Here's how the part is built. I have some questions about the finished solid (model axes, mm). A direction names the side the tool comes from. Coordinates: 2 decimals unless noted, no trailing zeros. Loops run counter-clockwise (first coordinate to the right, second up) from the corner with the lowest first, then second, coordinate; pieces in that order, holes last. Notation, with made-up numbers: M 54.25,56 L 68.25,56 A29 cw 68.25,87 Z; hole C 27.25,-13.75 d11. An arc over 180 degrees is marked long. Use CSV: the item, a comma, the result in double quotes. Start each with the question number.
Q1. Please list where these lines run through material, in increasing order: probe 1 along Y at (x, z) = (122, 3.05); probe 2 along Y at (x, z) = (144, 11); probe 3 along Y at (x, z) = (182, 16). Write a range as [from, to].
Q2. For pin 1 Ø4 at (y, z) = (91.5, 4) entering from +X; pin 2 Ø6.5 at (x, y) = (74, 48.5) entering from +Z; pin 3 Ø4 at (y, z) = (23.5, 3.5) entering from -X; pin 4 Ø3 at (y, z) = (23, 7) entering from +X, each with a flat end and sliding along its axis, tell me the tip position at first contact or that it passes through.
Q3. Which directions (+Z, -Z, +X, -X, +Y, -Y) give clear straight access to the entire face, cutting with the end or side of a thin tool? Please do faces 1 (the flat face through (243, 107, 4)), 2 (the flat face through (173, 29, 4)).
Q4. If we section it at B-B (x = 32): Please give me the cut outline in (y, z), and give its area (3 significant figures).
Q5. If we section it at A-A (x = 159): Please give me the cut outline in (y, z).
from build123d import *

# Parameters (mm, degrees)
F1_DEPTH = 4
F0_R     = 3
F0_R_2   = 2.5
F0_R_3   = 2
F0_R_4   = 12
F0_R_5   = 8
F2_DEPTH = 8
F3_DEPTH = 30


with BuildPart() as f1:
    # F0 (on Top) → F1 (new body)
    with BuildSketch(Plane.XY):
        with BuildLine():
            Line((236, 122), (236, 77))
            Line((236, 77), (249.9140349643, 77))
            Line((249.9140349643, 77), (286.1814989821, 119.8615483846))
            ThreePointArc((286.1814989821, 119.8615483846), (280.1803788328, 120.1541279906), (278.7929977309, 126))
            Line((278.7929977309, 126), (150, 126))
            Line((150, 126), (150, 122))
            Line((150, 122), (236, 122))
        make_face()
    extrude(amount=F1_DEPTH)



with BuildPart() as f1b:
    # F0 (on Top) → F1, piece 2 (new body)
    with BuildSketch(Plane.XY):
        Polygon((220.2986503489, 42), (243.1448041951, 69), (195, 69), (195, 42), align=None)
    extrude(amount=F1_DEPTH)


with BuildPart() as f1c:
    # F0 (on Top) → F1, piece 3 (new body)
    with BuildSketch(Plane.XY):
        Polygon((203.3755734259, 22), (215.221727272, 36), (177, 36), (177, 22), align=None)
    extrude(amount=F1_DEPTH)


with BuildPart() as f1d:
    # F0 (on Top) → F1, piece 4 (new body)
    with BuildSketch(Plane.XY):
        Polygon((188.1448041951, 4), (199.9909580413, 18), (177, 18), (177, 4), align=None)
    extrude(amount=F1_DEPTH)


with BuildPart() as f1e:
    # F0 (on Top) → F1, piece 5 (new body)
    with BuildSketch(Plane.XY):
        with BuildLine():
            Line((146, 10.582575695), (146, 119.417424305))
            ThreePointArc((146, 119.417424305), (140.4644660941, 120.4644660941), (139.417424305, 126))
            Line((139.417424305, 126), (10.582575695, 126))
            ThreePointArc((10.582575695, 126), (9.5355339059, 120.4644660941), (4, 119.417424305))
            Line((4, 119.417424305), (4, 10.582575695))
            ThreePointArc((4, 10.582575695), (9.5355339059, 9.5355339059), (10.582575695, 4))
            Line((10.582575695, 4), (139.417424305, 4))
            ThreePointArc((139.417424305, 4), (140.4644660941, 9.5355339059), (146, 10.582575695))
        make_face()
        with Locations((14, 23.5)):
            Circle(F0_R, mode=Mode.SUBTRACT)
        with Locations((26, 23.5)):
            Circle(F0_R, mode=Mode.SUBTRACT)
        with Locations((38, 23.5)):
            Circle(F0_R, mode=Mode.SUBTRACT)
        with Locations((50, 23.5)):
            Circle(F0_R, mode=Mode.SUBTRACT)
        with Locations((62, 23.5)):
            Circle(F0_R, mode=Mode.SUBTRACT)
        with Locations((74, 23.5)):
            Circle(F0_R, mode=Mode.SUBTRACT)
        with Locations((86, 23.5)):
            Circle(F0_R, mode=Mode.SUBTRACT)
        with Locations((98, 23.5)):
            Circle(F0_R, mode=Mode.SUBTRACT)
        with Locations((110, 23.5)):
            Circle(F0_R, mode=Mode.SUBTRACT)
        with Locations((122, 23.5)):
            Circle(F0_R, mode=Mode.SUBTRACT)
        with Locations((14, 38.5)):
            Circle(F0_R_2, mode=Mode.SUBTRACT)
        with Locations((26, 38.5)):
            Circle(F0_R_2, mode=Mode.SUBTRACT)
        with Locations((14, 48.5)):
            Circle(F0_R_2, mode=Mode.SUBTRACT)
        with Locations((26, 48.5)):
            Circle(F0_R_2, mode=Mode.SUBTRACT)
        with Locations((38, 38.5)):
            Circle(F0_R_2, mode=Mode.SUBTRACT)
        with Locations((50, 38.5)):
            Circle(F0_R_2, mode=Mode.SUBTRACT)
        with Locations((62, 38.5)):
            Circle(F0_R_2, mode=Mode.SUBTRACT)
        with Locations((74, 38.5)):
            Circle(F0_R_2, mode=Mode.SUBTRACT)
        with Locations((38, 48.5)):
            Circle(F0_R_2, mode=Mode.SUBTRACT)
        with Locations((50, 48.5)):
            Circle(F0_R_2, mode=Mode.SUBTRACT)
        with Locations((62, 48.5)):
            Circle(F0_R_2, mode=Mode.SUBTRACT)
        with Locations((74, 48.5)):
            Circle(F0_R_2, mode=Mode.SUBTRACT)
        with Locations((86, 38.5)):
            Circle(F0_R_2, mode=Mode.SUBTRACT)
        with Locations((98, 38.5)):
            Circle(F0_R_2, mode=Mode.SUBTRACT)
        with Locations((110, 38.5)):
            Circle(F0_R_2, mode=Mode.SUBTRACT)
        with Locations((86, 48.5)):
            Circle(F0_R_2, mode=Mode.SUBTRACT)
        with Locations((98, 48.5)):
            Circle(F0_R_2, mode=Mode.SUBTRACT)
        with Locations((110, 48.5)):
            Circle(F0_R_2, mode=Mode.SUBTRACT)
        with Locations((122, 38.5)):
            Circle(F0_R_2, mode=Mode.SUBTRACT)
        with Locations((122, 48.5)):
            Circle(F0_R_2, mode=Mode.SUBTRACT)
        with Locations((15, 96)):
            Circle(F0_R_3, mode=Mode.SUBTRACT)
        with Locations((34, 96)):
            Circle(F0_R_4, mode=Mode.SUBTRACT)
        with Locations((53, 96)):
            Circle(F0_R_3, mode=Mode.SUBTRACT)
        with Locations((99, 96)):
            Circle(F0_R_5, mode=Mode.SUBTRACT)
    extrude(amount=F1_DEPTH)


with BuildPart() as f1_1:
    add(f1.part)

    add(f1b.part)  # F2 merges F1b

    add(f1c.part)  # F2 merges F1c

    add(f1d.part)  # F2 merges F1d

    add(f1e.part)  # F2 merges F1e
    # F0 (on Top) → F2 (join)
    with BuildSketch(Plane.XY):
        Polygon((249.9140349643, 77), (236, 77), (150, 77), (150, 69), (195, 69), (243.1448041951, 69), align=None)
        with BuildLine():
            Line((150, 69), (150, 77))
            Line((150, 77), (150, 122))
            Line((150, 122), (150, 126))
            Line((150, 126), (148.582575695, 126))
            ThreePointArc((148.582575695, 126), (148.6545839116, 122.1738432132), (146, 119.417424305))
            Line((146, 119.417424305), (146, 10.582575695))
            ThreePointArc((146, 10.582575695), (148.6545839116, 7.8261567868), (148.582575695, 4))
            Line((148.582575695, 4), (150, 4))
            Line((150, 4), (150, 18))
            Line((150, 18), (150, 22))
            Line((150, 22), (150, 36))
            Line((150, 36), (150, 42))
            Line((150, 42), (150, 69))
        make_face()
        Polygon((195, 42), (150, 42), (150, 36), (173, 36), (173, 22), (150, 22), (150, 18), (173, 18), (173, 4), (177, 4), (177, 18), (199.9909580413, 18), (203.3755734259, 22), (177, 22), (177, 36), (215.221727272, 36), (220.2986503489, 42), align=None)
    extrude(amount=F2_DEPTH)

    # F0 (on Top) → F3 (join)
    with BuildSketch(Plane.XY):
        Polygon((0, 130), (0, 0), (190, 0), (300, 130), align=None)
        with Locations((6, 6)):
            Circle(F0_R_2, mode=Mode.SUBTRACT)
        with Locations((144, 6)):
            Circle(F0_R_2, mode=Mode.SUBTRACT)
        with BuildLine():
            Line((286.1814989821, 119.8615483846), (249.9140349643, 77))
            Line((249.9140349643, 77), (243.1448041951, 69))
            Line((243.1448041951, 69), (220.2986503489, 42))
            Line((220.2986503489, 42), (215.221727272, 36))
            Line((215.221727272, 36), (203.3755734259, 22))
            Line((203.3755734259, 22), (199.9909580413, 18))
            Line((199.9909580413, 18), (188.1448041951, 4))
            Line((188.1448041951, 4), (177, 4))
            Line((177, 4), (173, 4))
            Line((173, 4), (150, 4))
            Line((150, 4), (148.582575695, 4))
            ThreePointArc((148.582575695, 4), (148.6545839116, 7.8261567868), (146, 10.582575695))
            ThreePointArc((146, 10.582575695), (140.4644660941, 9.5355339059), (139.417424305, 4))
            Line((139.417424305, 4), (10.582575695, 4))
            ThreePointArc((10.582575695, 4), (9.5355339059, 9.5355339059), (4, 10.582575695))
            Line((4, 10.582575695), (4, 119.417424305))
            ThreePointArc((4, 119.417424305), (9.5355339059, 120.4644660941), (10.582575695, 126))
            Line((10.582575695, 126), (139.417424305, 126))
            ThreePointArc((139.417424305, 126), (140.4644660941, 120.4644660941), (146, 119.417424305))
            ThreePointArc((146, 119.417424305), (148.6545839116, 122.1738432132), (148.582575695, 126))
            Line((148.582575695, 126), (150, 126))
            Line((150, 126), (278.7929977309, 126))
            ThreePointArc((278.7929977309, 126), (280.1803788328, 120.1541279906), (286.1814989821, 119.8615483846))
        make_face(mode=Mode.SUBTRACT)
        with Locations((6, 124)):
            Circle(F0_R_2, mode=Mode.SUBTRACT)
        with Locations((144, 124)):
            Circle(F0_R_2, mode=Mode.SUBTRACT)
        with Locations((283.3755734259, 124)):
            Circle(F0_R_2, mode=Mode.SUBTRACT)
    extrude(amount=F3_DEPTH)


solid = f1_1.part
Results below:
1,probe 1,"[0, 20.5], [26.5, 36], [41, 46], [51, 130]"
1,probe 2,"[0, 3.5], [8.5, 11], [119, 121.5], [126.5, 130]"
1,probe 3,"[0, 4], [126, 130]"
2,pin 1,"x = 269.12"
2,pin 2,"z = 4"
2,pin 3,"x = 0"
2,pin 4,"x = 210.73"
3,face 1,"+Z"
3,face 2,"+Z, -Z"
4,outline,"M 0,0 L 84.17,0 L 84.17,4 L 4,4 L 4,30 L 0,30 Z; M 107.83,0 L 130,0 L 130,30 L 126,30 L 126,4 L 107.83,4 Z"
4,area,"633 mm^2"
5,outline,"M 0,0 L 4,0 L 4,30 L 0,30 Z; M 18,0 L 22,0 L 22,8 L 18,8 Z; M 36,0 L 42,0 L 42,8 L 36,8 Z; M 69,0 L 77,0 L 77,8 L 69,8 Z; M 122,0 L 130,0 L 130,30 L 126,30 L 126,4 L 122,4 Z"
